For this review, take the finished solid that the model builds, in its own axes (mm). A direction names the side the tool comes from. Round coordinates to 2 decimals unless told otherwise and drop trailing zeros. Order: outer loops, then holes, each group sorted by start corner. A loop starts at its lowest first (then second) coordinate and runs counter-clockwise, first axis right, second up. Notation, with made-up numbers: (41, -15.75) - (75, -15.75) arc R23 ccw to (75, 8.25) - close; hole circle Ø8 at (50, -29.75). An arc over 180 degrees is marked (long way). One line per item, written item: value.
```python
from build123d import *

# Parameters (mm, degrees)
BOSS_EXTRUDE1_DEPTH = 6.35
SKETCH2_R           = 2.286
CUT_EXTRUDE1_DEPTH  = 15.622107372
SKETCH3_W           = 4.572
SKETCH3_H           = 4.572
CUT_EXTRUDE2_DEPTH  = 7.62
SKETCH4_W           = 4.572
SKETCH4_H           = 4.572
CUT_EXTRUDE3_DEPTH  = 7.62
SKETCH5_R           = 2.794
SKETCH5_R_2         = 2.159
BOSS_EXTRUDE2_DEPTH = 7.62


with BuildPart() as part:
    # Sketch1 → Boss-Extrude1 (new body)
    with BuildSketch(Plane(origin=(0, 0, 0), x_dir=(1, 0, 0), z_dir=(0, 1, 0))):
        with BuildLine():
            Line((-2.032, -2.271845065), (-2.032, -10.16))
            Line((-2.032, -10.16), (-8.382, -10.16))
            Line((-8.382, -10.16), (-8.382, 10.16))
            Line((-8.382, 10.16), (-2.032, 10.16))
            Line((-2.032, 10.16), (-2.032, 2.271845065))
            ThreePointArc((-2.032, 2.271845065), (0, 3.048), (2.032, 2.271845065))
            Line((2.032, 2.271845065), (2.032, 10.16))
            Line((2.032, 10.16), (8.382, 10.16))
            Line((8.382, 10.16), (8.382, -10.16))
            Line((8.382, -10.16), (2.032, -10.16))
            Line((2.032, -10.16), (2.032, -2.271845065))
            ThreePointArc((2.032, -2.271845065), (0, -3.048), (-2.032, -2.271845065))
        make_face()
    extrude(amount=-BOSS_EXTRUDE1_DEPTH)

    # Sketch2 → Cut-Extrude1 (cut, through all)
    with BuildSketch(Plane(origin=(0, 0, 0), x_dir=(1, 0, 0), z_dir=(0, 1, 0))):
        with Locations(Location((0, 0, 0), (0, 0, 270))):
            Circle(SKETCH2_R)
    extrude(amount=-CUT_EXTRUDE1_DEPTH, mode=Mode.SUBTRACT)

    # Sketch3 → Cut-Extrude2 (cut)
    with BuildSketch(Plane.XY.offset(10.16)):
        with Locations((-5.207, -3.175)):
            Rectangle(SKETCH3_W, SKETCH3_H)
        with Locations((5.207, -3.175)):
            Rectangle(SKETCH3_W, SKETCH3_H)
    extrude(amount=-CUT_EXTRUDE2_DEPTH, mode=Mode.SUBTRACT)

    # Sketch4 → Cut-Extrude3 (cut)
    with BuildSketch(Plane(origin=(0, 0, -10.16), x_dir=(-1, 0, 0), z_dir=(0, 0, -1))):
        with Locations((-5.207, -3.175)):
            Rectangle(SKETCH4_W, SKETCH4_H)
        with Locations((5.207, -3.175)):
            Rectangle(SKETCH4_W, SKETCH4_H)
    extrude(amount=-CUT_EXTRUDE3_DEPTH, mode=Mode.SUBTRACT)

    # Sketch5 → Boss-Extrude2 (add)
    # profile 1 of 4: a face of its own
    with BuildSketch(Plane(origin=(0, 0, 0), x_dir=(1, 0, 0), z_dir=(0, 1, 0))):
        with Locations(Location((-5.207, -5.08, 0), (0, 0, 90))):
            Circle(SKETCH5_R)
        with Locations(Location((-5.207, -5.08, 0), (0, 0, 90))):
            Circle(SKETCH5_R_2, mode=Mode.SUBTRACT)
    # profile 2 of 4: a face of its own
    with BuildSketch(Plane(origin=(0, 0, 0), x_dir=(1, 0, 0), z_dir=(0, 1, 0))):
        with Locations(Location((-5.207, 5.08, 0), (0, 0, 90))):
            Circle(SKETCH5_R)
        with Locations(Location((-5.207, 5.08, 0), (0, 0, 90))):
            Circle(SKETCH5_R_2, mode=Mode.SUBTRACT)
    # profile 3 of 4: a face of its own
    with BuildSketch(Plane(origin=(0, 0, 0), x_dir=(1, 0, 0), z_dir=(0, 1, 0))):
        with Locations(Location((5.207, 5.08, 0), (0, 0, 90))):
            Circle(SKETCH5_R)
        with Locations(Location((5.207, 5.08, 0), (0, 0, 90))):
            Circle(SKETCH5_R_2, mode=Mode.SUBTRACT)
    # profile 4 of 4: a face of its own
    with BuildSketch(Plane(origin=(0, 0, 0), x_dir=(1, 0, 0), z_dir=(0, 1, 0))):
        with Locations(Location((5.207, -5.08, 0), (0, 0, 90))):
            Circle(SKETCH5_R)
        with Locations(Location((5.207, -5.08, 0), (0, 0, 90))):
            Circle(SKETCH5_R_2, mode=Mode.SUBTRACT)
    extrude(amount=BOSS_EXTRUDE2_DEPTH)


solid = part.part
```
Item 1: Take a section at C-C (y = 5.25). Write out the cut boundary in (x, z), plus the area to 3 significant figures.
Returned:
outline: circle Ø5.59 at (-5.21, -5.08); circle Ø5.59 at (-5.21, 5.08); circle Ø5.59 at (5.21, -5.08); circle Ø5.59 at (5.21, 5.08); hole circle Ø4.32 at (-5.21, -5.08); hole circle Ø4.32 at (-5.21, 5.08); hole circle Ø4.32 at (5.21, -5.08); hole circle Ø4.32 at (5.21, 5.08)
area: 39.5 mm^2
Item 2: The part is to be moulded in two halves that separate along X. For faces 1 (the flat face through (2.032, -3, 6)), 2 (the flat face through (-8, -3, -10.16)), say which applies: +X half, -X half, draft (parallel to the pull), parting line (faces both ways), or undercut.
Returned:
face 1: undercut
face 2: draft
Item 3: Take a section at A-A (x = 0). Write out the cut boundary in (y, z).
Returned:
outline: (-6.35, -3.05) - (0, -3.05) - (0, -2.29) - (-6.35, -2.29) - close; (-6.35, 2.29) - (0, 2.29) - (0, 3.05) - (-6.35, 3.05) - close
Item 4: For P1, Ø1.3, axis at x = -5, z = -6, coming from the +Y side; P2, Ø2.5, axis at x = 4.5, y = -4, coming from the +Z side; P3, Ø6, axis at y = 4, z = 5.5, coming from the +X side, all flat-tipped, find the tip position at first contact; note any pin that passes through.
Returned:
P1: y = 0
P2: z = 2.54
P3: x = 8
Item 5: Machinability: for faces 3 (the flat face through (-7.493, -3, 6)), 4 (the flat face through (-5, -0.889, -6)), 5 (the cylindrical face through (-6.67, 3.76, -3.49)), which of the approach directions +Z, -Z, +X, -X, +Y, -Y give a long, thin tool a straight path to every point of the face, cutting with its end or side? Answer none if there is none.
Returned:
face 3: +Z
face 4: -Z
face 5: +Y
Item 6: Take a section at D-D (z = 0). Write out the cut boundary in (x, y).
Returned:
outline: (-8.38, -6.35) - (-2.29, -6.35) - (-2.29, 0) - (-8.38, 0) - close; (2.29, -6.35) - (8.38, -6.35) - (8.38, 0) - (2.29, 0) - close
Item 7: Take a section at B-B (z = -5.08). Count the separate pieces of the cut face and the enclosed holes in it, plus the area to 3 significant figures.
Returned:
separate pieces: 2
enclosed holes: 2
area: 58.2 mm^2
Item 8: Wall thickness on line 1 (X direction, y = 2.5, z = 5.08); line 2 (X direction, y = -3.5, z = -7.5); line 3 (Z direction, x = 5.25, y = 2.25): over which ranges is each line inside the solid? List them lowest first.
Returned:
line 1: -8 to -7.37, -3.05 to -2.41, 2.41 to 3.05, 7.37 to 8
line 2: -8.38 to -7.49, -2.92 to -2.03, 2.03 to 2.92, 7.49 to 8.38
line 3: -7.87 to -7.24, -2.92 to -2.29, 2.29 to 2.92, 7.24 to 7.87
